```python
from build123d import *

# Parameters (mm, degrees)
BOSS_EXTRUDE1_DEPTH      = 500
BOSS_EXTRUDE1_DEPTH_BACK = 500
LPATTERN1_COUNT          = 17
LPATTERN1_PITCH          = 60
SKETCH6_W                = 111
SKETCH6_H                = 2.7
CUT_EXTRUDE1_DEPTH       = 501.102489496


with BuildPart() as part:
    # Sketch5 → Boss-Extrude1 (new, two sides: drawn at the far end of the back side and taken through both)
    with BuildSketch(Plane(origin=(0, 0, 0), x_dir=(0, 0, -1), z_dir=(1, 0, 0)).offset(-BOSS_EXTRUDE1_DEPTH_BACK)):
        with BuildLine():
            Line((-8.499999996, -2.75), (8.499999996, -2.75))
            Line((8.499999996, -2.75), (8.499999996, 2.25))
            ThreePointArc((8.499999996, 2.25), (8.353553387, 2.603553391), (7.999999996, 2.75))
            Line((7.999999996, 2.75), (5.299999996, 2.75))
            Line((5.299999996, 2.75), (5.299999996, 1.55))
            Line((5.299999996, 1.55), (7.299999998, 1.55))
            Line((7.299999998, 1.55), (7.299999998, 0.05))
            Line((7.299999998, 0.05), (4.249999998, 0.05))
            Line((4.249999998, 0.05), (3.749999998, -0.45))
            Line((3.749999998, -0.45), (0.499999998, -0.45))
            Line((0.499999998, -0.45), (0, -0.738675133))
            Line((0, -0.738675133), (-0.499999998, -0.45))
            Line((-0.499999998, -0.45), (-3.749999998, -0.45))
            Line((-3.749999998, -0.45), (-4.249999998, 0.05))
            Line((-4.249999998, 0.05), (-7.299999998, 0.05))
            Line((-7.299999998, 0.05), (-7.299999998, 1.55))
            Line((-7.299999998, 1.55), (-5.299999996, 1.55))
            Line((-5.299999996, 1.55), (-5.299999996, 2.75))
            Line((-5.299999996, 2.75), (-7.999999996, 2.75))
            ThreePointArc((-7.999999996, 2.75), (-8.353553387, 2.603553391), (-8.499999996, 2.25))
            Line((-8.499999996, 2.25), (-8.499999996, -2.75))
        make_face()
    extrude(amount=BOSS_EXTRUDE1_DEPTH + BOSS_EXTRUDE1_DEPTH_BACK)

    # Sketch3 → Cut-Revolve1 (revolve, cut)
    with BuildSketch(Plane.XY, mode=Mode.PRIVATE) as cut_revolve1_sk:
        Polygon((-483.25, -0.45), (-483.25, -1.75), (-481.75, -1.75), (-481.75, -2.75), (-480, -2.75), (-480, -0.45), align=None)
    cut_revolve1 = revolve(cut_revolve1_sk.sketch.rotate(Axis((-480, -2.75, 0), (0, 1, 0)), 180), axis=Axis((-480, -2.75, 0), (0, 1, 0)), mode=Mode.SUBTRACT)

    # LPattern1: Cut-Revolve1 ×17
    with Locations(*[(i * LPATTERN1_PITCH, 0, 0) for i in range(1, LPATTERN1_COUNT)]):
        add(cut_revolve1, mode=Mode.SUBTRACT)

    # Sketch6 → Cut-Extrude1 (cut, through all)
    with BuildSketch(Plane(origin=(0, 2.75, 0), x_dir=(1, 0, 0), z_dir=(0, 1, 0))):
        Polygon((389, 126.212542349), (389, 8.499999996), (389, 7.999999996), (500, 7.999999996), (500, 5.299999996), (389, 5.299999996), (389, -102.065679631), (557.848580128, -102.065679631), (557.848580128, 126.212542349), align=None)
        with Locations((444.5, 6.649999996)):
            Rectangle(SKETCH6_W, SKETCH6_H)
    extrude(amount=-CUT_EXTRUDE1_DEPTH, mode=Mode.SUBTRACT)


solid = part.part
```
Read the model definition and answer for the solid it produces. Units are mm, in the model's axes. Coordinates: 2 decimals unless noted, no trailing zeros. Write each loop counter-clockwise with the first axis right and the second up, starting at its lowest first coordinate (ties: lowest second). Pieces come first, ordered by that corner, then holes. Notation, with made-up numbers: (55.25, -9.5) -> (87.25, -9.5) arc R10 cw to (87.25, -0.5) -> close; hole circle Ø6 at (-9, 65). An arc over 180 degrees is marked (long way). Return JSON: item names as keys, results as strings.
1. Find the intervals of material crossed by line 1 along Y through (x, z) = (-150.5, 6); line 2 along Z through (x, y) = (-180, -2.5); line 3 along Z through (x, y) = (178, 1.35), in increasing order. Write a range as from..to.
Found:
{"line 1": "-2.75..0.05, 1.55..2.75", "line 2": "-8.5..-1.75, 1.75..8.5", "line 3": "-8.5..-7.3, 7.3..8.5"}
2. A cutting plane is placed at A-A (x = 220). Determine the outline of the cut face in (y, z).
Found:
{"outline": "(-2.75, -8.5) -> (2.25, -8.5) arc R0.5 ccw to (2.75, -8) -> (2.75, -5.3) -> (1.55, -5.3) -> (1.55, -7.3) -> (0.05, -7.3) -> (0.05, -4.25) -> (-0.45, -3.75) -> (-0.45, -0.5) -> (-0.74, 0) -> (-0.45, 0.5) -> (-0.45, 3.75) -> (0.05, 4.25) -> (0.05, 7.3) -> (1.55, 7.3) -> (1.55, 5.3) -> (2.75, 5.3) -> (2.75, 8) arc R0.5 ccw to (2.25, 8.5) -> (-2.75, 8.5) -> close"}
3. Each of these flat-tipped pins is pushed along its axis until it touches: P1, Ø3, axis at x = 300, z = 0, coming from the -Y side; P2, Ø7, axis at x = 119, z = 0, coming from the +Y side; P3, Ø2, axis at x = -58.5, z = 0.5, coming from the +Y side; P4, Ø7, axis at x = 1, z = 1.5, coming from the +Y side. Where does it stop, or does it pass through?
Found:
{"P1": "through", "P2": "y = -0.45", "P3": "y = -1.75", "P4": "y = 0.05"}
